from build123d import *

# Parameters (mm, degrees)
SKETCH1_W           = 4.5
SKETCH1_H           = 19.5
CUT_EXTRUDE1_DEPTH  = 2.2
SKETCH5_R           = 1.6
CUT_EXTRUDE2_DEPTH  = 21.512191497
CUT_EXTRUDE3_START  = -7
CUT_EXTRUDE3_DEPTH  = 2.65
BOSS_EXTRUDE1_START = -2.2
SKETCH2_3_R         = 6
SKETCH2_3_R_2       = 4.5
BOSS_EXTRUDE1_DEPTH = 15.1


with BuildPart() as part:
    # Sketch1 → Revolve1 (revolve)
    with BuildSketch(Plane.XY, mode=Mode.PRIVATE) as revolve1_sk:
        with Locations((2.25, 0)):
            Rectangle(SKETCH1_W, SKETCH1_H)
    revolve(revolve1_sk.sketch.rotate(Axis((0, 9.75, 0), (0, -1, 0)), 180), axis=Axis((0, 9.75, 0), (0, -1, 0)))

    # Sketch2 → Cut-Extrude1 (cut)
    with BuildSketch(Plane(origin=(0, 9.75, 0), x_dir=(1, 0, 0), z_dir=(0, 1, 0))):
        with BuildLine():
            Line((-2.9, -3.440930107), (-2.9, 3.440930107))
            ThreePointArc((-2.9, 3.440930107), (-4.5, 0), (-2.9, -3.440930107))
        make_face()
        with BuildLine():
            ThreePointArc((4.5, 0), (4.080441153, 1.897366596), (2.9, 3.440930107))
            Line((2.9, 3.440930107), (2.9, -3.440930107))
            ThreePointArc((2.9, -3.440930107), (4.080441153, -1.897366596), (4.5, 0))
        make_face()
    cut_extrude1 = extrude(amount=-CUT_EXTRUDE1_DEPTH, mode=Mode.SUBTRACT)

    # Sketch5 → Cut-Extrude2 (cut, through all)
    with BuildSketch(Plane(origin=(0, 9.75, 0), x_dir=(1, 0, 0), z_dir=(0, 1, 0))):
        with Locations(Location((0, 0, 0), (0, 0, 180))):
            Circle(SKETCH5_R)
    cut_extrude2 = extrude(amount=-CUT_EXTRUDE2_DEPTH, mode=Mode.SUBTRACT)

    # Sketch6 → Cut-Extrude3 (cut)
    with BuildSketch(Plane(origin=(0, 9.75, 0), x_dir=(1, 0, 0), z_dir=(0, 1, 0)).offset(CUT_EXTRUDE3_START)):
        Polygon((3.406366588, 0), (1.703183294, 2.95), (-1.703183294, 2.95), (-1.703183294, -2.95), (1.703183294, -2.95), align=None)
        Polygon((-1.703183294, -2.95), (-1.703183294, 2.95), (-3.406366588, 0), align=None)
    cut_extrude3 = extrude(amount=CUT_EXTRUDE3_DEPTH, mode=Mode.SUBTRACT)

    # Mirror2: Cut-Extrude1, Cut-Extrude2, Cut-Extrude3 across plane
    add(cut_extrude1.mirror(Plane.ZX), mode=Mode.SUBTRACT)
    add(cut_extrude2.mirror(Plane.ZX), mode=Mode.SUBTRACT)
    add(cut_extrude3.mirror(Plane.ZX), mode=Mode.SUBTRACT)

    # Sketch2<3> → Boss-Extrude1 (add)
    with BuildSketch(Plane(origin=(0, 9.75, 0), x_dir=(1, 0, 0), z_dir=(0, 1, 0)).offset(BOSS_EXTRUDE1_START)):
        with Locations(Location((0, 0, 0), (0, 0, 180))):
            Circle(SKETCH2_3_R)
        Circle(SKETCH2_3_R_2, mode=Mode.SUBTRACT)
    extrude(amount=-BOSS_EXTRUDE1_DEPTH)


solid = part.part
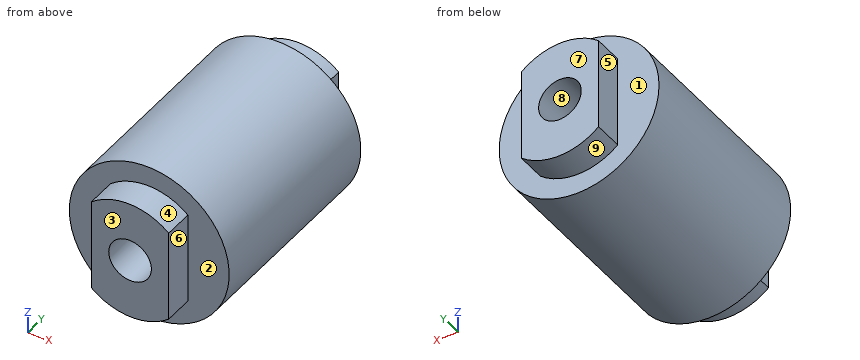
Could you check a few things on this model? Use its own coordinates, in mm. Face numbers are marked on the shaded views. A direction names the side the tool comes from. Coordinates: 2 decimals unless noted, no trailing zeros. Write each loop counter-clockwise with the first axis right and the second up, starting at its lowest first coordinate (ties: lowest second). Pieces come first, ordered by that corner, then holes. Notation, with made-up numbers: (64, 56) - (73, 56) arc R21 ccw to (73, 67) - close; hole circle Ø7 at (44.5, -39.75). An arc over 180 degrees is marked (long way). Put each result on its own line as item: value. Start each with the question number.
Q1. Which directions (+Z, -Z, +X, -X, +Y, -Y) give clear straight access to the entire face, cutting with the end or side of a thin tool? Please do the marked faces 1, 2, 3, 4 and 5.
Q2. Please list where these lines run through material, in increasing order: L1, parallel to Y at x = 0.75, z = -2.5; L2, parallel to Z at x = 0, y = -6.45; L3, parallel to Y at x = -3, z = 1.
Q3. I want a section at D-D on z = 3.75. Write out the boundary of the cut face in (x, y).
Q4. I want a section at A-A on y = -4.25. Write out the boundary of the cut face in (x, z), plus the area to 3 significant figures.
Q5. I'm going to push flat-ended pins straight in: P1, Ø1.1, axis at y = 8, z = -1, coming from the -X side; P2, Ø1, axis at y = 5.5, z = 3, coming from the -X side; P3, Ø1.8, axis at y = -8.5, z = 0.5, coming from the -X side. Where does each tip first touch, or does it pass through?
Q6. Thinking about a two-plate mould opening in X: for the marked faces 6, 7, 8 and 9, which applies, pulls with the +X half, pulls with the -X half, needs draft (parallel to the pull), parting line crosses it, or undercut?
Checks:
1. face 1: +Y
1. face 2: -Y
1. face 3: +Z, -Z, +X, -X, -Y
1. face 4: +Z, -Y
1. face 5: +Z, -Z, -X, +Y
2. L1: -9.75 to -5.4, -2.75 to 2.75, 5.4 to 9.75
2. L2: -6 to -1.6, 1.6 to 6
2. L3: -7.55 to 7.55
3. outline: (-4.68, -7.55) - (-2.49, -7.55) - (-2.49, -9.75) - (2.49, -9.75) - (2.49, -7.55) - (4.68, -7.55) - (4.68, 7.55) - (2.49, 7.55) - (2.49, 9.75) - (-2.49, 9.75) - (-2.49, 7.55) - (-4.68, 7.55) - close
4. outline: circle Ø12 at (0, 0); hole (-3.41, 0) - (-1.7, -2.95) - (1.7, -2.95) - (3.41, 0) - (1.7, 2.95) - (-1.7, 2.95) - close
4. area: 83.0 mm²
5. P1: x = -5.96
5. P2: x = -5.45
5. P3: x = -2.9
6. face 6: pulls with the +X half
6. face 7: needs draft
6. face 8: undercut
6. face 9: parting line crosses it
